Source: CAD feature listing. Evaluate the final solid. Frame: model axes, mm. A direction names the side the tool comes from. Give positions to 0.01 mm unless a question says otherwise; leave off trailing zeros. Write each loop counter-clockwise with the first axis right and the second up, starting at its lowest first coordinate (ties: lowest second). Pieces come first, ordered by that corner, then holes. Notation, with made-up numbers: M -27.5,-21.75 L 28.5,-21.75 A25 cw 28.5,-4.75 Z; hole C 43,14.5 d7. An arc over 180 degrees is marked long. Use CSV: the item, a comma, the result in double quotes. Start each with the question number.
from build123d import *

# Parameters (mm, degrees)
F0_W      = 39.37
F0_H      = 39.37
F1_DEPTH  = 26.2128
F2_W      = 39.37
F2_H      = 7.112
F3_DEPTH  = 40.291659534
F4_W      = 27.94
F4_H      = 32.004
F5_DEPTH  = 25.4
F6_DEPTH  = 0.762
F7_DEPTH  = 0.6096
F9_DEPTH  = 7.62
F11_DEPTH = 7.62


with BuildPart() as f1:
    # F0 (on Top) → F1 (new body)
    with BuildSketch(Plane.XY):
        with BuildLine():
            Line((-19.685, -22.225), (19.685, -22.225))
            ThreePointArc((19.685, -22.225), (21.4810512242, -21.4810512242), (22.225, -19.685))
            Line((22.225, -19.685), (22.225, 19.685))
            ThreePointArc((22.225, 19.685), (21.4810512242, 21.4810512242), (19.685, 22.225))
            Line((19.685, 22.225), (-19.685, 22.225))
            ThreePointArc((-19.685, 22.225), (-20.4412358464, 22.1098107853), (-21.1288809737, 21.7746908225))
            ThreePointArc((-21.1288809737, 21.7746908225), (-21.4448596213, 21.5165278085), (-21.7154231521, 21.211100201))
            ThreePointArc((-21.7154231521, 21.211100201), (-22.0942400053, 20.4894641675), (-22.225, 19.685))
            Line((-22.225, 19.685), (-22.225, -19.685))
            ThreePointArc((-22.225, -19.685), (-21.4810512242, -21.4810512242), (-19.685, -22.225))
        make_face()
        Rectangle(F0_W, F0_H, mode=Mode.SUBTRACT)
    extrude(amount=F1_DEPTH)

    # F2 (on face) → F3 (join)
    with BuildSketch(Plane(origin=(0, -19.685, 0), x_dir=(-1, 0, 0), z_dir=(0, 1, 0))):
        with Locations((0, 22.6568)):
            Rectangle(F2_W, F2_H)
    extrude(amount=F3_DEPTH)

    # F4 (on face) → F5 (cut)
    with BuildSketch(Plane(origin=(0, 0, 19.1008), x_dir=(1, 0, 0), z_dir=(0, 0, -1))):
        Rectangle(F4_W, F4_H)
    extrude(amount=-F5_DEPTH, mode=Mode.SUBTRACT)

    # F6 (cut): a face of the model
    f6_faces = [f1.faces().sort_by_distance(p)[0] for p in [
        (0, -21.5963820715, 26.2128),
    ]]
    extrude(f6_faces, amount=-F6_DEPTH, mode=Mode.SUBTRACT)

    # F7 (add): a face of the model
    f7_faces = [f1.faces().sort_by_distance(p)[0] for p in [
        (0, -21.5963820715, 0),
    ]]
    extrude(f7_faces, amount=F7_DEPTH)

    # F8 (on face) → F9 (cut)
    with BuildSketch(Plane(origin=(0, -19.685, 0), x_dir=(-1, 0, 0), z_dir=(0, 1, 0))):
        with BuildLine():
            ThreePointArc((0, 11.7856), (-2.54, 9.2456), (0, 6.7056))
            Line((0, 6.7056), (0, 11.7856))
        make_face()
        with BuildLine():
            Line((0, 11.7856), (0, 6.7056))
            ThreePointArc((0, 6.7056), (1.7960512242, 7.4495487758), (2.54, 9.2456))
            ThreePointArc((2.54, 9.2456), (1.7960512242, 11.0416512242), (0, 11.7856))
        make_face()
    extrude(amount=-F9_DEPTH, mode=Mode.SUBTRACT)

    # F10 (on face) → F11 (cut)
    with BuildSketch(Plane.XZ.offset(-19.685)):
        with BuildLine():
            ThreePointArc((0, 11.7856), (-2.54, 9.2456), (0, 6.7056))
            Line((0, 6.7056), (0, 11.7856))
        make_face()
        with BuildLine():
            Line((0, 11.7856), (0, 6.7056))
            ThreePointArc((0, 6.7056), (1.7960512242, 7.4495487758), (2.54, 9.2456))
            ThreePointArc((2.54, 9.2456), (1.7960512242, 11.0416512242), (0, 11.7856))
        make_face()
    extrude(amount=-F11_DEPTH, mode=Mode.SUBTRACT)


solid = f1.part
Item 1: Set-up query: faces 5 (the flat face through (-22.225, 0, 13)), 6 (the flat face through (13.97, 0, 22)), 7 (the flat face through (-17, 0, 19.101)). Return all of +Z, -Z, +X, -X, +Y, -Y with unobstructed straight access to the full face (end or side cutting, diameter ignored); none if empty.
Item 2: Section C-C (y = 3). Return the cut outline in (x, z) (3 decimals), plus the area to 3 significant figures.
Item 3: Contact query for a flat-ended pin moving along its axis: pin 1 Ø1.5 at (x, y) = (-12, -1) entering from +Z (3 decimals). Output: stop coordinate, or through.
Item 4: Material intervals for probe 1 along Y at (x, z) = (-16, 18) (3 decimals); probe 2 along X at (y, z) = (11, 22.5) (3 decimals), sorted ascending.
Item 5: Pull-direction query (Y, two-part tool) for faces 1 (the cylindrical face through (-21.5, -21.46, 12.6)), 2 (the flat face through (-19.685, 0, 9)), 3 (the flat face through (22.225, 0, 13)), 4 (the flat face through (0, 22.225, 13)); classes: released by +Y, released by -Y, zero draft, split by the parting line, or undercut.
Item 6: Section A-A (x = -11.5). Return the cut outline in (y, z) (3 decimals).
Item 7: Section D-D (z = 12.5). Return the cut outline in (x, y) (3 decimals), plus the area to 3 significant figures.
Item 8: Section B-B (z = 21.5). Return the cut outline in (x, y) (3 decimals), plus the area to 3 significant figures.
Output values:
1,face 5,"+Z, -Z, -X, +Y, -Y"
1,face 6,"+Z, -Z"
1,face 7,"-Z"
2,outline,"M -22.225,-0.61 L -19.685,-0.61 L -19.685,19.101 L -13.97,19.101 L -13.97,25.451 L -22.225,25.451 Z; M 13.97,19.101 L 19.685,19.101 L 19.685,-0.61 L 22.225,-0.61 L 22.225,25.451 L 13.97,25.451 Z"
2,area,"205 mm2"
3,pin 1,"passes through"
4,probe 1,"y = -22.225 to -19.685, 19.685 to 22.225"
4,probe 2,"x = -22.225 to -13.97, 13.97 to 22.225"
5,face 1,"released by -Y"
5,face 2,"undercut"
5,face 3,"zero draft"
5,face 4,"released by +Y"
6,outline,"M -22.225,-0.61 L -19.685,-0.61 L -19.685,19.101 L -16.002,19.101 L -16.002,25.451 L -22.225,25.451 Z; M 16.002,19.101 L 19.685,19.101 L 19.685,-0.61 L 22.225,-0.61 L 22.225,25.451 L 16.002,25.451 Z"
7,outline,"M -22.225,-19.685 A2.54 ccw -19.685,-22.225 L 19.685,-22.225 A2.54 ccw 22.225,-19.685 L 22.225,19.685 A2.54 ccw 19.685,22.225 L -19.685,22.225 A2.54 ccw -22.225,19.685 Z; hole M -19.685,-19.685 L 19.685,-19.685 L 19.685,19.685 L -19.685,19.685 Z"
7,area,"420 mm2"
8,outline,"M -22.225,-19.685 A2.54 ccw -19.685,-22.225 L 19.685,-22.225 A2.54 ccw 22.225,-19.685 L 22.225,19.685 A2.54 ccw 19.685,22.225 L -19.685,22.225 A2.54 ccw -22.225,19.685 Z; hole M -13.97,-16.002 L 13.97,-16.002 L 13.97,16.002 L -13.97,16.002 Z"
8,area,"1,080 mm2"
